from build123d import *
from build123d import SkipClean  # not in build123d's __all__

# Parameters (mm, degrees)
F2_R          = 0.5
F3_DEPTH      = 4.251
F3_DEPTH_BACK = 4.251
F4_R          = 0.5
F5_DEPTH      = 4.2510001
F5_DEPTH_BACK = 4.2510001
F7_DEPTH      = 7.2
F8_SIZE2      = 0.5
F8_SIZE       = 0.5


with BuildPart() as f1:
    # F0 (on Front) → F1 (revolve)
    with BuildSketch(Plane.XZ):
        Polygon((0.75, 1), (0.75, 0), (2.75, 0), (2.75, 1.7), (4.25, 5.7), (4.25, 9.2), (2.9, 9.2), (2.9, 5.2), (0.75, 6.4413030788), (0.75, 2.7505553499), (0.1, 2.375277675), (0.1, 1.375277675), align=None)
    revolve(axis=Axis((0, 0, 4.6), (0, 0, -1)))

    # F2 (on Front) → F3 (cut, two sides)
    with BuildSketch(Plane.XZ) as f3_sk:
        with Locations((0, 3.7)):
            Circle(F2_R)
    extrude(amount=-F3_DEPTH, mode=Mode.SUBTRACT)
    extrude(f3_sk.sketch, amount=F3_DEPTH_BACK, mode=Mode.SUBTRACT)

    # F4 (on Right) → F5 (cut, two sides)
    with BuildSketch(Plane.YZ) as f5_sk:
        with Locations((0, 3.7)):
            Circle(F4_R)
    extrude(amount=-F5_DEPTH, mode=Mode.SUBTRACT)
    extrude(f5_sk.sketch, amount=F5_DEPTH_BACK, mode=Mode.SUBTRACT)

    # F6 (on Top) → F7 (cut)
    with BuildSketch(Plane.XY):
        with BuildLine():
            ThreePointArc((2.6516504294, 3.3587572106), (3.1943648253, 4.0460926544), (3.5628585232, 4.8405618624))
            ThreePointArc((3.5628585232, 4.8405618624), (1.875, 5.7104618903), (0, 6.0104076401))
            Line((0, 6.0104076401), (2.6516504294, 3.3587572106))
        make_face()
        with BuildLine():
            ThreePointArc((1.2201895167, 2.464475105), (1.9868873303, 2.8300336469), (2.6516504294, 3.3587572106))
            Line((2.6516504294, 3.3587572106), (0, 6.0104076401))
            ThreePointArc((0, 6.0104076401), (-1.875, 5.7104618903), (-3.5628585232, 4.8405618624))
            ThreePointArc((-3.5628585232, 4.8405618624), (-2.6703621866, 3.3776019518), (-1.2201895167, 2.464475105))
            ThreePointArc((-1.2201895167, 2.464475105), (0, 2.75), (1.2201895167, 2.464475105))
        make_face()
        with BuildLine():
            ThreePointArc((-3.5628585232, -4.8405618624), (0, -6.0104076401), (3.5628585232, -4.8405618624))
            ThreePointArc((3.5628585232, -4.8405618624), (2.6703621866, -3.3776019518), (1.2201895167, -2.464475105))
            ThreePointArc((1.2201895167, -2.464475105), (0, -2.75), (-1.2201895167, -2.464475105))
            ThreePointArc((-1.2201895167, -2.464475105), (-2.6703621866, -3.3776019518), (-3.5628585232, -4.8405618624))
        make_face()
        with BuildLine():
            ThreePointArc((-4.8405618624, 3.5628585232), (-6.0104076401, 0), (-4.8405618624, -3.5628585232))
            ThreePointArc((-4.8405618624, -3.5628585232), (-3.3776019518, -2.6703621866), (-2.464475105, -1.2201895167))
            ThreePointArc((-2.464475105, -1.2201895167), (-2.75, 0), (-2.464475105, 1.2201895167))
            ThreePointArc((-2.464475105, 1.2201895167), (-3.3776019518, 2.6703621866), (-4.8405618624, 3.5628585232))
        make_face()
        with BuildLine():
            Line((3.3587572106, 2.6516504294), (6.0104076401, 0))
            ThreePointArc((6.0104076401, 0), (5.7104618903, 1.875), (4.8405618624, 3.5628585232))
            ThreePointArc((4.8405618624, 3.5628585232), (4.0460926544, 3.1943648253), (3.3587572106, 2.6516504294))
        make_face()
        with BuildLine():
            ThreePointArc((4.8405618624, -3.5628585232), (5.7104618903, -1.875), (6.0104076401, 0))
            Line((6.0104076401, 0), (3.3587572106, 2.6516504294))
            ThreePointArc((3.3587572106, 2.6516504294), (2.8300336469, 1.9868873303), (2.464475105, 1.2201895167))
            ThreePointArc((2.464475105, 1.2201895167), (2.6776675054, 0.626575399), (2.75, 0))
            ThreePointArc((2.75, 0), (2.6776675054, -0.626575399), (2.464475105, -1.2201895167))
            ThreePointArc((2.464475105, -1.2201895167), (3.3776019518, -2.6703621866), (4.8405618624, -3.5628585232))
        make_face()
    with SkipClean():  # cleaning this boolean's faces spoils the solid; the shape is the same uncleaned
        extrude(amount=F7_DEPTH, mode=Mode.SUBTRACT)

    # F8
    f8_edges = [f1.edges().sort_by_distance(p)[0] for p in [
        (-4.25, 0, 9.2),
    ]]
    chamfer(f8_edges, length=F8_SIZE, length2=F8_SIZE2)


solid = f1.part
Input: part model. Units: mm. Frame: model coordinates. A direction names the side the tool comes from. Round coordinates to 2 decimals unless told otherwise and drop trailing zeros. Write each loop counter-clockwise with the first axis right and the second up, starting at its lowest first coordinate (ties: lowest second). Pieces come first, ordered by that corner, then holes.
1) Cut plane C-C (z = 1.25). Return the cut outline in (x, y).
2) Cut plane A-A (z = 3.5). Count the separate pieces of the cut face and the enclosed holes in it, then the cut area to 3 significant figures.
3) Contact query for flat-ended pins moving along their axis: P1, Ø2, axis at x = -1.5, z = 1.5, coming from the +Y side; P2, Ø1.4, axis at x = -3.5, y = -1, coming from the -Z side; P3, Ø1.5, axis at y = 0.5, z = 1, coming from the -X side. Output: stop coordinate, or through.
4) Draft query along Z for faces 4 (the flat face through (0, -3.4, 7.2)), 5 (the cylindrical face through (-1.6, -0.5, 3.7)), 6 (the cylindrical face through (-0.75, -0.03, 0.49)), 7 (the cylindrical face through (-0.5, 1.6, 3.7)). Return one class per face: pulls with the +Z half, pulls with the -Z half, needs draft (parallel to the pull), parting line crosses it, or undercut.
5) Reachability of faces 1 (the cylindrical face through (-1.82, 2.73, 5.02)), 2 (the cylindrical face through (-2.72, 1.8, 5.02)), 3 (the cylindrical face through (-0.098, -0.744, 4.98)) from +Z, -Z, +X, -X, +Y, -Y: full face, straight path, thin tool, end or side. Return the list, or none.
6) Ray query, L1, parallel to Y at x = 0, z = 0.65; L2, parallel to Y at x = 1.4, z = 3.7; L3, parallel to X at y = 0, z = 7.6. Return the intervals inside material, ascending.
Geometry says:
1. outline: circle Ø5.5 at (0, 0); hole circle Ø0.63 at (0, 0)
2. separate pieces: 4
2. enclosed holes: 0
2. area: 18.5 mm2
3. P1: stops at y = 2.7
3. P2: stops at z = 7.2
3. P3: stops at x = -2.75
4. face 4: pulls with the -Z half
4. face 5: undercut
4. face 6: needs draft
4. face 7: undercut
5. face 1: -Z, +Y
5. face 2: -Z, -X
5. face 3: +Z
6. L1: y = -2.75 to -0.75, 0.75 to 2.75
6. L2: y = -2.53 to -0.5, 0.5 to 2.53
6. L3: x = -4.25 to -2.9, 2.9 to 4.25
